from build123d import *

# Parameters (mm, degrees)
F1_DEPTH = 82


with BuildPart() as f1:
    # F0 (on Right) → F1 (new body)
    with BuildSketch(Plane.YZ):
        with BuildLine():
            Line((17.505096594, 69.6115375847), (31.005096594, 69.6115375847))
            ThreePointArc((31.005096594, 69.6115375847), (21.459155048, 73.5655960386), (17.505096594, 83.1115375847))
            Line((17.505096594, 83.1115375847), (17.505096594, 69.6115375847))
        make_face()
        with BuildLine():
            ThreePointArc((17.505096594, 13.7115375847), (21.459155048, 23.2574791307), (31.005096594, 27.2115375847))
            Line((31.005096594, 27.2115375847), (17.505096594, 27.2115375847))
            Line((17.505096594, 27.2115375847), (17.505096594, 13.7115375847))
        make_face()
        with BuildLine():
            Line((31.005096594, 0.2115375847), (31.005096594, 3.2115375847))
            ThreePointArc((31.005096594, 3.2115375847), (23.5804753915, 6.2869163822), (20.505096594, 13.7115375847))
            Line((20.505096594, 13.7115375847), (17.505096594, 13.7115375847))
            ThreePointArc((17.505096594, 13.7115375847), (21.459155048, 4.1655960386), (31.005096594, 0.2115375847))
        make_face()
        with BuildLine():
            ThreePointArc((20.505096594, 13.7115375847), (23.5804753915, 21.1361587871), (31.005096594, 24.2115375847))
            Line((31.005096594, 24.2115375847), (31.005096594, 27.2115375847))
            ThreePointArc((31.005096594, 27.2115375847), (21.459155048, 23.2574791307), (17.505096594, 13.7115375847))
            Line((17.505096594, 13.7115375847), (20.505096594, 13.7115375847))
        make_face()
        with BuildLine():
            Line((44.505096594, 13.7115375847), (41.505096594, 13.7115375847))
            ThreePointArc((41.505096594, 13.7115375847), (38.4297177964, 6.2869163822), (31.005096594, 3.2115375847))
            Line((31.005096594, 3.2115375847), (31.005096594, 0.2115375847))
            ThreePointArc((31.005096594, 0.2115375847), (40.55103814, 4.1655960386), (44.505096594, 13.7115375847))
        make_face()
        with BuildLine():
            ThreePointArc((31.005096594, 96.6115375847), (21.459155048, 92.6574791307), (17.505096594, 83.1115375847))
            Line((17.505096594, 83.1115375847), (20.505096594, 83.1115375847))
            ThreePointArc((20.505096594, 83.1115375847), (31.005096594, 93.6115375847), (41.505096594, 83.1115375847))
            Line((41.505096594, 83.1115375847), (44.505096594, 83.1115375847))
            ThreePointArc((44.505096594, 83.1115375847), (40.55103814, 92.6574791307), (31.005096594, 96.6115375847))
        make_face()
        with BuildLine():
            ThreePointArc((17.505096594, 83.1115375847), (21.459155048, 73.5655960386), (31.005096594, 69.6115375847))
            Line((31.005096594, 69.6115375847), (31.005096594, 72.6115375847))
            ThreePointArc((31.005096594, 72.6115375847), (23.5804753915, 75.6869163822), (20.505096594, 83.1115375847))
            Line((20.505096594, 83.1115375847), (17.505096594, 83.1115375847))
        make_face()
        with BuildLine():
            Line((44.505096594, 27.2115375847), (44.505096594, 13.7115375847))
            ThreePointArc((44.505096594, 13.7115375847), (40.55103814, 4.1655960386), (31.005096594, 0.2115375847))
            Line((31.005096594, 0.2115375847), (36.8288183167, 0.1773171395))
            ThreePointArc((36.8288183167, 0.1773171395), (58.1558844242, 8.901363301), (67.005096594, 30.1767992345))
            Line((67.005096594, 30.1767992345), (67.005096594, 66.6115375847))
            ThreePointArc((67.005096594, 66.6115375847), (58.2183000296, 87.8247410203), (37.005096594, 96.6115375847))
            Line((37.005096594, 96.6115375847), (31.005096594, 96.6115375847))
            ThreePointArc((31.005096594, 96.6115375847), (40.55103814, 92.6574791307), (44.505096594, 83.1115375847))
            Line((44.505096594, 83.1115375847), (44.505096594, 69.6115375847))
            Line((44.505096594, 69.6115375847), (63.005096594, 69.6115375847))
            Line((63.005096594, 69.6115375847), (63.005096594, 27.2115375847))
            Line((63.005096594, 27.2115375847), (44.505096594, 27.2115375847))
        make_face()
        with BuildLine():
            ThreePointArc((31.005096594, 27.2115375847), (40.55103814, 23.2574791307), (44.505096594, 13.7115375847))
            Line((44.505096594, 13.7115375847), (44.505096594, 27.2115375847))
            Line((44.505096594, 27.2115375847), (31.005096594, 27.2115375847))
        make_face()
        with BuildLine():
            ThreePointArc((31.005096594, 24.2115375847), (38.4297177964, 21.1361587871), (41.505096594, 13.7115375847))
            Line((41.505096594, 13.7115375847), (44.505096594, 13.7115375847))
            ThreePointArc((44.505096594, 13.7115375847), (40.55103814, 23.2574791307), (31.005096594, 27.2115375847))
            Line((31.005096594, 27.2115375847), (31.005096594, 24.2115375847))
        make_face()
        with BuildLine():
            ThreePointArc((44.505096594, 83.1115375847), (40.55103814, 73.5655960386), (31.005096594, 69.6115375847))
            Line((31.005096594, 69.6115375847), (44.505096594, 69.6115375847))
            Line((44.505096594, 69.6115375847), (44.505096594, 83.1115375847))
        make_face()
        with BuildLine():
            Line((31.005096594, 72.6115375847), (31.005096594, 69.6115375847))
            ThreePointArc((31.005096594, 69.6115375847), (40.55103814, 73.5655960386), (44.505096594, 83.1115375847))
            Line((44.505096594, 83.1115375847), (41.505096594, 83.1115375847))
            ThreePointArc((41.505096594, 83.1115375847), (38.4297177964, 75.6869163822), (31.005096594, 72.6115375847))
        make_face()
    extrude(amount=F1_DEPTH)


solid = f1.part
Verification items for the finished model (mm, model axes). A direction names the side the tool comes from. Give positions to 0.01 mm unless a question says otherwise; leave off trailing zeros. Write each loop counter-clockwise with the first axis right and the second up, starting at its lowest first coordinate (ties: lowest second). Pieces come first, ordered by that corner, then holes. Notation, with made-up numbers: M -10.5,77 L 1.5,77 A20 cw 1.5,110 Z; hole C 49,15 d7. An arc over 180 degrees is marked long. Put each result on its own line as item: value. Start each with the question number.
1. Scan lines: line 1 along Z through (x, y) = (36, 38); line 2 along Z through (x, y) = (13, 25); line 3 along Y through (x, z) = (64.5, 55.5). Record each from-to range of solid material in increasing order. Write a range as [from, to].
2. Section check B-B (z = 87). Record the cut outline in (x, y), and give its area (3 significant figures).
3. Draft check along Z on faces 3 (the face through (40.43, 57.92, 8.67)), 4 (the face through (40.43, 58.45, 87.59)), 5 (the face through (40, 40, 69.612)), 6 (the face through (40, 17.505, 21)). Enter one of: +Z half, -Z half, draft (parallel to the pull), parting line (faces both ways), or undercut.
4. Section check C-C (x = 67). Record the cut outline in (y, z), and give its area (3 significant figures).
5. Section check A-A (y = 55.5). Record the cut outline in (x, z).
6. Set-up check for faces 1 (the face through (40, 63.005, 49)), 2 (the face through (40, 34, 96.612)): record each of +Z, -Z, +X, -X, +Y, -Y from which the full face is reachable in a straight line by a thin tool's end or side.
7. Section check D-D (y = 35). Record the cut outline in (x, z), and give its area (3 significant figures).
8. Go/stop test with flat-tipped pins: pin 1 Ø8 at (x, y) = (27, 41.5) entering from -Z; pin 2 Ø2 at (x, y) = (14, 49) entering from -Z; pin 3 Ø1.5 at (x, y) = (20.5, 46.5) entering from +Z; pin 4 Ø12 at (y, z) = (31.5, 13.5) entering from -X. Record where each tip stops, or that it passes through.
Answer list:
1. line 1: [0.19, 5.88], [21.54, 27.21], [69.61, 75.28], [90.94, 96.6]
1. line 2: [1.62, 5.1], [22.32, 27.21], [69.61, 74.5], [91.72, 95.2]
1. line 3: [63.01, 67.01]
2. outline: M 0,18.08 L 82,18.08 L 82,21.25 L 0,21.25 Z; M 0,40.76 L 82,40.76 L 82,59.01 L 0,59.01 Z
2. area: 1,760 mm2
3. face 3: -Z half
3. face 4: +Z half
3. face 5: undercut
3. face 6: draft
4. outline: M 17.51,13.71 A13.5 ccw 31.01,0.21 L 36.83,0.18 A30 ccw 67.01,30.18 L 67.01,66.61 A30 ccw 37.01,96.61 L 31.01,96.61 A13.5 ccw 17.51,83.11 L 17.51,69.61 L 63.01,69.61 L 63.01,27.21 L 17.51,27.21 Z; hole C 31.01,13.71 d21; hole C 31.01,83.11 d21
4. area: 1,690 mm2
5. outline: M 0,6.56 L 82,6.56 L 82,27.21 L 0,27.21 Z; M 0,69.61 L 82,69.61 L 82,90.23 L 0,90.23 Z
6. face 1: +X, -X, -Y
6. face 2: +Z, +X, -X, +Y, -Y
7. outline: M 0,0.19 L 82,0.19 L 82,4 L 0,4 Z; M 0,23.42 L 82,23.42 L 82,27.21 L 0,27.21 Z; M 0,69.61 L 82,69.61 L 82,73.4 L 0,73.4 Z; M 0,92.82 L 82,92.82 L 82,96.61 L 0,96.61 Z
7. area: 1,240 mm2
8. pin 1: z = 0.18
8. pin 2: z = 2.26
8. pin 3: z = 95.31
8. pin 4: through
